Autodesk Fusion 360 part; units mm, degrees
sketch "Sketch1" plane through (0, 0, 0) normal (0, 0, 1) x (1, 0, 0)
  line L0 (12, -12) -> (-12, -12)
  line L1 (-12, -12) -> (-12, 12)
  line L2 (-12, 12) -> (12, 12)
  line L3 (12, 12) -> (12, -12)
  line L4 (12, -12) -> (-12, 12) construction
  line L5 (-12, -12) -> (12, 12) construction
  dimension "d1" = 24
  dimension "d2" = 24
extrude "Extrude1" add sketch "Sketch1" along normal blind 3
sketch "Sketch2" plane through (0, 0, 3) normal (0, 0, 1) x (-1, 0, 0)
  line L0 (-12, -12) -> (12, -12)
  line L1 (12, -12) -> (12, 12)
  line L2 (12, 12) -> (-12, 12)
  line L3 (-12, 12) -> (-12, -12)
  circle A0 centre (10, -10) radius 1.1
  circle A1 centre (-10, -10) radius 1.1
  circle A2 centre (10, 10) radius 1.1
  circle A3 centre (-10, 10) radius 1.1
  dimension "d5" = 2.2
  dimension "d6" = 2.2
  dimension "d7" = 2.2
  dimension "d8" = 2.2
  dimension "d9" = 10
  dimension "d10" = 10
  dimension "d11" = 10
  dimension "d12" = 10
  dimension "d13" = 10
  dimension "d14" = 10
  dimension "d15" = 10
  dimension "d16" = 10
extrude "Extrude2" cut sketch "Sketch2" against normal through all contours A0 | A1 | A2 | A3
sketch "Sketch3" plane through (0, 0, 3) normal (0, 0, 1) x (-1, 0, 0)
  circle A0 centre (10, -10) radius 1.1
  circle A1 centre (10, 10) radius 1.1
  circle A2 centre (-10, -10) radius 1.1
  circle A3 centre (-10, 10) radius 1.1
  line L0 (-12, -12) -> (12, -12)
  line L1 (12, -12) -> (12, 12)
  line L2 (12, 12) -> (-12, 12)
  line L3 (-12, 12) -> (-12, -12)
  circle A4 centre (0, 0) radius 6
  dimension "d18" = 12
extrude "Extrude3" cut sketch "Sketch3" against normal blind 6 contours A4
sketch "Sketch4" plane through (0, 0, 3) normal (0, 0, 1) x (-1, 0, 0)
  circle A0 centre (0, 0) radius 6
  circle A1 centre (10, -10) radius 1.1
  circle A2 centre (10, 10) radius 1.1
  circle A3 centre (-10, -10) radius 1.1
  circle A4 centre (-10, 10) radius 1.1
  line L0 (-12, -12) -> (12, -12)
  line L1 (12, -12) -> (12, 12)
  line L2 (12, 12) -> (-12, 12)
  line L3 (-12, 12) -> (-12, -12)
  circle A5 centre (10, -10) radius 1.2
  circle A6 centre (-10, -10) radius 1.2
  circle A7 centre (10, 10) radius 1.2
  circle A8 centre (-10, 10) radius 1.2
  dimension "d21" = 2.4
  dimension "d22" = 2.4
  dimension "d23" = 2.4
  dimension "d24" = 2.4
extrude "Extrude4" cut sketch "Sketch4" against normal blind 5 contours A5 | A6 | A7 | A8
Geometry check sheet. Reference: the model listing, model coordinates, mm. Coordinates: 2 decimals unless noted, no trailing zeros. Order: outer loops, then holes, each group sorted by start corner. A loop starts at its lowest first (then second) coordinate and runs counter-clockwise, first axis right, second up.
Item 1: Scan lines: line 1 along X through (y, z) = (-10, 0.6); line 2 along X through (y, z) = (0, 2.15). Record each from-to range of solid material in increasing order.
Item 2: Mould release check, pull along X, two halves, no side actions. Record for faces 1 (the flat face through (12, 0, 1)), 2 (the cylindrical face through (-9.74, -8.83, 1.52)), 3 (the cylindrical face through (9.446, -8.935, 1.521)), 4 (the flat face through (-6, 3, 0)): released by +X, released by -X, zero draft, split by the parting line, or undercut.
Item 3: Section check B-B (y = 10). Enter the section's corners in (x, z).
Item 4: Section check A-A (x = 0). Enter the section's corners in (y, z).
Check sheet entries:
1. line 1: x = -12 to -11.2, -8.8 to 8.8, 11.2 to 12
1. line 2: x = -12 to -6, 6 to 12
2. face 1: released by +X
2. face 2: undercut
2. face 3: undercut
2. face 4: zero draft
3. outline: (-12, 0) - (-11.2, 0) - (-11.2, 3) - (-12, 3) - close; (-8.8, 0) - (8.8, 0) - (8.8, 3) - (-8.8, 3) - close; (11.2, 0) - (12, 0) - (12, 3) - (11.2, 3) - close
4. outline: (-12, 0) - (-6, 0) - (-6, 3) - (-12, 3) - close; (6, 0) - (12, 0) - (12, 3) - (6, 3) - close
